Geometry check sheet. Reference: the model listing, model coordinates, mm. Coordinates: 2 decimals unless noted, no trailing zeros. Order: outer loops, then holes, each group sorted by start corner. A loop starts at its lowest first (then second) coordinate and runs counter-clockwise, first axis right, second up. Notation, with made-up numbers: (-31.75, 73) - (-2.75, 73) arc R25 ccw to (-2.75, 91) - close; hole circle Ø8 at (77.25, 34.5). An arc over 180 degrees is marked (long way). Return JSON: item names as keys, results as strings. Group by question number.
Item 1: Section check B-B on x = -35. Enter the section's corners in (y, z), then the cut area to 3 significant figures.
Item 2: Draft check along X on faces 1 (the cylindrical face through (36.582, 0.351, -0.089)), 2 (the flat face through (0.6, 6.35, 4.3)), 3 (the flat face through (-40, 0, 0)). Enter one of: pulls with the +X half, pulls with the -X half, needs draft (parallel to the pull), parting line crosses it, or undercut.
Item 3: Scan lines: probe 1 along Y at (x, z) = (-20, -3.5); probe 2 along Y at (x, z) = (35, -2.5); probe 3 along X at (y, z) = (0, 0.5). Record each from-to range of solid material in increasing order.
Item 4: Section check A-A on z = 0. Enter the section's corners in (x, y), then the cut area to 3 significant figures.
Item 5: Section check C-C on x = 35. Enter the section's corners in (y, z).
Item 6: Section check D-D on y = -4.75. Enter the section's corners in (x, z), then the cut area to 3 significant figures.
Autodesk Inventor part; units mm, degrees
ref_plane "YZ Plane" through (0, 0, 0) normal (1, 0, 0) x (0, 1, 0)
ref_plane "XZ Plane" through (0, 0, 0) normal (0, 1, 0) x (-1, 0, 0)
ref_plane "XY Plane" through (0, 0, 0) normal (0, 0, 1) x (1, 0, 0)
sketch "スケッチ1" plane through (0, 0, 0) normal (0, 1, 0) x (-1, 0, 0)
  line L0 (-40, 6.35) -> (40, 6.35)
  line L1 (40, 6.35) -> (40, -6.35)
  line L2 (40, -6.35) -> (-40, -6.35)
  line L3 (-40, -6.35) -> (-40, 6.35)
  line L4 (-40, 6.35) -> (40, -6.35) construction
  line L5 (40, 6.35) -> (-40, -6.35) construction
  arc A0 (0, 3.3541) -> (0, -3.3541) centre (-3, 0) ccw
  line L6 (-40, 0) -> (0, 0) construction
  line L7 (0, 6.35) -> (0, -6.35) construction
  arc A1 (0, -3.3541) -> (0, 3.3541) centre (3, 0) ccw
  point P0 (0, -3.3541)
  dimension "d0" = 80
  dimension "d1" = 12.7
  dimension "d2" = 9
  dimension "d3" = 3
extrude "押し出し1" add sketch "スケッチ1" along normal mid plane 12.7
sketch "スケッチ2" plane through (-40, 6.35, 6.35) normal (0, 0, 1) x (1, 0, 0)
  line L0 (80, -12.7) -> (80, 0)
  line L1 (80, -6.35) -> (0, -6.35) construction
  line L2 (0, -12.7) -> (0, 0)
  line L3 (80, 0) -> (0, 0)
  line L4 (40, 0) -> (40, -12.7) construction
  line L5 (80, -12.7) -> (0, -12.7)
  point P0 (40, -6.35)
  point P1 (75, -6.35)
  point P2 (60, -6.35)
  point P3 (20, -6.35)
  point P4 (5, -6.35)
  dimension "d6" = 15
  dimension "d7" = 15
  dimension "d8" = 40
hole "穴1" at (35, 0, 6.35) at (20, 0, 6.35) direction (0, 0, -1) diameter 3.242 end through all
hole "穴2" at (-20, 0, 6.35) at (-35, 0, 6.35) direction (0, 0, -1) diameter 4.134 end through all
properties part number "SC133-20kg"
Computed:
{
 "1": {"outline": "(-6.35, -6.35) - (-2.07, -6.35) - (-2.07, 6.35) - (-6.35, 6.35) - close; (2.07, -6.35) - (6.35, -6.35) - (6.35, 6.35) - (2.07, 6.35) - close", "area": "109 mm²"},
 "2": {"face 1": "undercut", "face 2": "needs draft", "face 3": "pulls with the -X half"},
 "3": {"probe 1": "y = -6.35 to -2.07, 2.07 to 6.35", "probe 2": "y = -6.35 to -1.62, 1.62 to 6.35", "probe 3": "x = -40 to -37.07, -32.93 to -22.07, -17.93 to -7.47, 7.47 to 18.38, 21.62 to 33.38, 36.62 to 40"},
 "4": {"outline": "(-40, -6.35) - (-7.5, -6.35) - (-7.5, 6.35) - (-40, 6.35) - close; (7.5, -6.35) - (40, -6.35) - (40, 6.35) - (7.5, 6.35) - close; hole circle Ø4.13 at (-35, 0); hole circle Ø4.13 at (-20, 0); hole circle Ø3.24 at (20, 0); hole circle Ø3.24 at (35, 0)", "area": "782 mm²"},
 "5": {"outline": "(-6.35, -6.35) - (-1.62, -6.35) - (-1.62, 6.35) - (-6.35, 6.35) - close; (1.62, -6.35) - (6.35, -6.35) - (6.35, 6.35) - (1.62, 6.35) - close"},
 "6": {"outline": "(-40, -6.35) - (40, -6.35) - (40, 6.35) - (-40, 6.35) - close; hole (0, -3.35) arc R4.5 ccw (long way) to (0, 3.35) arc R4.5 ccw (long way) to start", "area": "903 mm²"}
}
